Source: CAD feature listing. Evaluate the final solid. Frame: model axes, mm. Face numbers are marked on the shaded views. A direction names the side the tool comes from. Coordinates: 2 decimals unless noted, no trailing zeros. Write each loop counter-clockwise with the first axis right and the second up, starting at its lowest first coordinate (ties: lowest second). Pieces come first, ordered by that corner, then holes. Notation, with made-up numbers: (-20.75, -15) - (31.25, -15) arc R7 ccw to (31.25, -11) - close; hole circle Ø3 at (4, 31.5). An arc over 180 degrees is marked (long way). One line per item, written item: value.
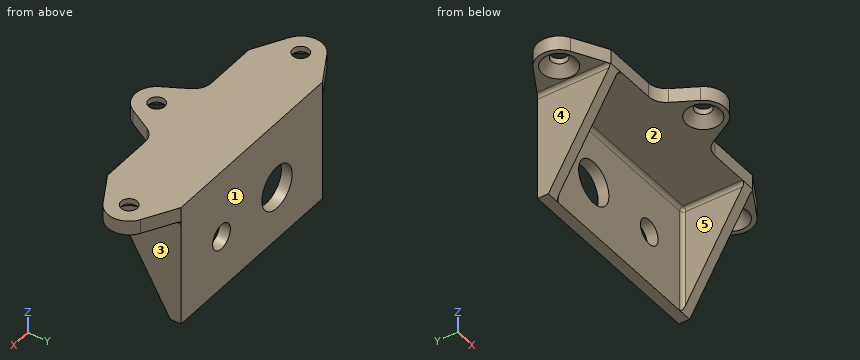
from build123d import *

# Parameters (mm, degrees)
SKETCH1_W                                       = 50
SKETCH1_H                                       = 30
SKETCH1_R                                       = 6
SKETCH1_R_2                                     = 3.5
BOSS_EXTRUDE1_DEPTH                             = 3
SKETCH2_W                                       = 50
SKETCH2_H                                       = 20.5
BOSS_EXTRUDE2_DEPTH                             = 4
BOSS_EXTRUDE3_DEPTH                             = 3
BOSS_EXTRUDE4_START                             = -50
BOSS_EXTRUDE4_DEPTH                             = 3
BOSS_EXTRUDE5_DEPTH                             = 4
CSK_FOR_M4_FLAT_HEAD_MACHINE_SCREW1_D           = 4.5
CSK_FOR_M4_FLAT_HEAD_MACHINE_SCREW1_DEPTH       = 10
CSK_FOR_M4_FLAT_HEAD_MACHINE_SCREW1_CSINK_D     = 9.4
CSK_FOR_M4_FLAT_HEAD_MACHINE_SCREW1_CSINK_ANGLE = 90
CSK_FOR_M4_FLAT_HEAD_MACHINE_SCREW1_TIP         = 1.351936393
FILLET1_R                                       = 5
FILLET2_R                                       = 1


with BuildPart() as part:
    # Sketch1 → Boss-Extrude1 (new body)
    with BuildSketch(Plane(origin=(0, 0, 0), x_dir=(1, 0, 0), z_dir=(0, 1, 0))):
        Rectangle(SKETCH1_W, SKETCH1_H)
        with Locations(Location((-10, 0, 0), (0, 0, 270))):
            Circle(SKETCH1_R, mode=Mode.SUBTRACT)
        with Locations(Location((12, 0, 0), (0, 0, 270))):
            Circle(SKETCH1_R_2, mode=Mode.SUBTRACT)
    extrude(amount=BOSS_EXTRUDE1_DEPTH)

    # Sketch2 → Boss-Extrude2 (add)
    with BuildSketch(Plane.XY.offset(15)):
        with Locations((0, -7.25)):
            Rectangle(SKETCH2_W, SKETCH2_H)
    extrude(amount=BOSS_EXTRUDE2_DEPTH)

    # Sketch3 → Boss-Extrude3 (add)
    with BuildSketch(Plane.ZY.offset(25)):
        Polygon((-15, 3), (-15, 0), (15, -17.5), (19, -17.5), (19, 3), align=None)
    extrude(amount=BOSS_EXTRUDE3_DEPTH)

    # Sketch3<2> → Boss-Extrude4 (add)
    with BuildSketch(Plane.ZY.offset(25).offset(BOSS_EXTRUDE4_START)):
        Polygon((-15, 3), (-15, 0), (15, -17.5), (19, -17.5), (19, 3), align=None)
    extrude(amount=-BOSS_EXTRUDE4_DEPTH)

    # Sketch5 → Boss-Extrude5 (add)
    with BuildSketch(Plane.XY.offset(19)):
        with BuildLine():
            Line((-28, 3), (-36.937527692, -2.018276473))
            ThreePointArc((-36.937527692, -2.018276473), (-40, -7.25), (-36.937527692, -12.481723527))
            Line((-36.937527692, -12.481723527), (-28, -17.5))
            Line((-28, -17.5), (-28, 3))
        make_face()
        with BuildLine():
            Line((28, 3), (36.937527692, -2.018276473))
            ThreePointArc((36.937527692, -2.018276473), (40, -7.25), (36.937527692, -12.481723527))
            Line((36.937527692, -12.481723527), (28, -17.5))
            Line((28, -17.5), (28, 3))
        make_face()
        with BuildLine():
            Line((10.25, -17.5), (-10.25, -17.5))
            Line((-10.25, -17.5), (-5.231723527, -26.437527692))
            ThreePointArc((-5.231723527, -26.437527692), (0, -29.5), (5.231723527, -26.437527692))
            Line((5.231723527, -26.437527692), (10.25, -17.5))
        make_face()
    extrude(amount=-BOSS_EXTRUDE5_DEPTH)

    # CSK for M4 Flat Head Machine Screw1
    with Locations(Plane(origin=(0, 0, 15), x_dir=(-1, 0, 0), z_dir=(0, 0, -1))):
        with Locations((-34, -7.25), (34, -7.25), (0, -23.5)):
            CounterSinkHole(CSK_FOR_M4_FLAT_HEAD_MACHINE_SCREW1_D / 2, CSK_FOR_M4_FLAT_HEAD_MACHINE_SCREW1_CSINK_D / 2, depth=CSK_FOR_M4_FLAT_HEAD_MACHINE_SCREW1_DEPTH, counter_sink_angle=CSK_FOR_M4_FLAT_HEAD_MACHINE_SCREW1_CSINK_ANGLE)
            with Locations((0, 0, -(CSK_FOR_M4_FLAT_HEAD_MACHINE_SCREW1_DEPTH + CSK_FOR_M4_FLAT_HEAD_MACHINE_SCREW1_TIP / 2))):  # 118° drill point
                Cone(0, CSK_FOR_M4_FLAT_HEAD_MACHINE_SCREW1_D / 2, CSK_FOR_M4_FLAT_HEAD_MACHINE_SCREW1_TIP, mode=Mode.SUBTRACT)

    # Fillet1
    fillet1_edges = [part.edges().sort_by_distance(p)[0] for p in [
        (-10.25, -17.5, 17),
        (10.25, -17.5, 17),
    ]]
    fillet(fillet1_edges, radius=FILLET1_R)

    # Fillet2
    # the kernel refuses this fillet: 1 mm, written as the material it adds along each edge
    with BuildSketch(Plane(origin=(-24, -1, 14), x_dir=(0, 1, 0), z_dir=(0, 0, 1))) as fillet2_piece_1_section:
        Polygon((0, 0), (FILLET2_R, 0), (FILLET2_R, FILLET2_R), (0, FILLET2_R), align=None)
    fillet2_piece_1 = extrude(amount=FILLET2_R, mode=Mode.PRIVATE)
    fillet2_piece_1 = fillet2_piece_1 - Plane(origin=(-24, -1, 14), x_dir=(0.7071067811865475, -0.7071067811865475, 0), z_dir=(0, 0, 1)) * Sphere(FILLET2_R, mode=Mode.PRIVATE)
    add(fillet2_piece_1)
    with BuildSketch(Plane(origin=(24, -1, 14), x_dir=(1, 0, 0), z_dir=(0, 0, 1))) as fillet2_piece_2_section:
        Polygon((0, 0), (FILLET2_R, 0), (FILLET2_R, FILLET2_R), (0, FILLET2_R), align=None)
    fillet2_piece_2 = extrude(amount=FILLET2_R, mode=Mode.PRIVATE)
    fillet2_piece_2 = fillet2_piece_2 - Plane(origin=(24, -1, 14), x_dir=(-0.7071067811865475, -0.7071067811865475, 0), z_dir=(0, 0, 1)) * Sphere(FILLET2_R, mode=Mode.PRIVATE)
    add(fillet2_piece_2)
    with BuildSketch(Plane(origin=(-25, -17.5, 15), x_dir=(1, 0, 0), z_dir=(0, 1, 0))) as fillet2_piece_3_section:
        with BuildLine():
            CenterArc((FILLET2_R, FILLET2_R), FILLET2_R, 180, 90)
            Line((0, FILLET2_R), (0, 0))
            Line((0, 0), (FILLET2_R, 0))
        make_face()
    fillet2_piece_3 = extrude(amount=16.5, mode=Mode.PRIVATE)
    fillet2_piece_3 = split(fillet2_piece_3, bisect_by=Plane(origin=(-24.77263385, -15.290921561, 11.213008391), z_dir=(0, 0.8637789008984336, 0.5038710255240861)), keep=Keep.TOP, mode=Mode.PRIVATE)
    add(fillet2_piece_3)
    with BuildSketch(Plane(origin=(25, -1, 15), x_dir=(-1, 0, 0), z_dir=(0, -1, 0))) as fillet2_piece_4_section:
        with BuildLine():
            CenterArc((FILLET2_R, FILLET2_R), FILLET2_R, 180, 90)
            Line((0, FILLET2_R), (0, 0))
            Line((0, 0), (FILLET2_R, 0))
        make_face()
    fillet2_piece_4 = extrude(amount=16.5, mode=Mode.PRIVATE)
    fillet2_piece_4 = split(fillet2_piece_4, bisect_by=Plane(origin=(24.77263385, -15.290921561, 11.213008391), z_dir=(0, 0.8637789008984336, 0.5038710255240861)), keep=Keep.TOP, mode=Mode.PRIVATE)
    add(fillet2_piece_4)
    with BuildSketch(Plane(origin=(24, 0, 15), x_dir=(0, -1, 0), z_dir=(-1, 0, 0))) as fillet2_piece_5:
        with BuildLine():
            CenterArc((FILLET2_R, -FILLET2_R), FILLET2_R, 90, 90)
            Line((0, -FILLET2_R), (0, 0))
            Line((0, 0), (FILLET2_R, 0))
        make_face()
    extrude(amount=48)
    with BuildSketch(Plane(origin=(-25, 0, 14), x_dir=(1, 0, 0), z_dir=(0, 0, -1))) as fillet2_piece_6_section:
        with BuildLine():
            CenterArc((FILLET2_R, FILLET2_R), FILLET2_R, 180, 90)
            Line((0, FILLET2_R), (0, 0))
            Line((0, 0), (FILLET2_R, 0))
        make_face()
    fillet2_piece_6 = extrude(amount=29, mode=Mode.PRIVATE)
    fillet2_piece_6 = split(fillet2_piece_6, bisect_by=Plane(origin=(-24.77197237, -6.451381469, -3.94048891), z_dir=(0, 0.8637789008984336, 0.5038710255240861)), keep=Keep.TOP, mode=Mode.PRIVATE)
    add(fillet2_piece_6)
    with BuildSketch(Plane(origin=(25, 0, -15), x_dir=(0, -1, 0), z_dir=(0, 0, 1))) as fillet2_piece_7_section:
        with BuildLine():
            CenterArc((FILLET2_R, -FILLET2_R), FILLET2_R, 90, 90)
            Line((0, -FILLET2_R), (0, 0))
            Line((0, 0), (FILLET2_R, 0))
        make_face()
    fillet2_piece_7 = extrude(amount=29, mode=Mode.PRIVATE)
    fillet2_piece_7 = split(fillet2_piece_7, bisect_by=Plane(origin=(24.77197237, -6.451381469, -3.94048891), z_dir=(0, 0.8637789008984336, 0.5038710255240861)), keep=Keep.TOP, mode=Mode.PRIVATE)
    add(fillet2_piece_7)
    with BuildSketch(Plane(origin=(-28, -20, 15), x_dir=(0, 0, -1), z_dir=(0, 1, 0))) as fillet2_piece_8_section:
        with BuildLine():
            CenterArc((FILLET2_R, FILLET2_R), FILLET2_R, 180, 90)
            Line((0, FILLET2_R), (0, 0))
            Line((0, 0), (FILLET2_R, 0))
        make_face()
    fillet2_piece_8 = extrude(amount=23, mode=Mode.PRIVATE)
    fillet2_piece_8 = split(fillet2_piece_8, bisect_by=Plane(origin=(-28.224621948, -14.787732132, 10.350397941), z_dir=(0, 0.8637789008984336, 0.5038710255240861)), keep=Keep.TOP, mode=Mode.PRIVATE)
    fillet2_piece_8 = split(fillet2_piece_8, bisect_by=Plane(origin=(-32.565520465, -14.936534495, 14.773416923), z_dir=(0.48958794860434196, 0.8719539211342491, 0)), keep=Keep.TOP, mode=Mode.PRIVATE)
    fillet2_piece_8 = split(fillet2_piece_8, bisect_by=Plane(origin=(-32.527453001, 0.457908757, 14.773416923), z_dir=(0.48958794860434235, -0.8719539211342491, 0)), keep=Keep.TOP, mode=Mode.PRIVATE)
    add(fillet2_piece_8)
    with BuildSketch(Plane(origin=(28, -20, 15), x_dir=(1, 0, 0), z_dir=(0, 1, 0))) as fillet2_piece_9_section:
        with BuildLine():
            CenterArc((FILLET2_R, FILLET2_R), FILLET2_R, 180, 90)
            Line((0, FILLET2_R), (0, 0))
            Line((0, 0), (FILLET2_R, 0))
        make_face()
    fillet2_piece_9 = extrude(amount=23, mode=Mode.PRIVATE)
    fillet2_piece_9 = split(fillet2_piece_9, bisect_by=Plane(origin=(32.565520464, -14.936534495, 14.773416923), z_dir=(-0.48958794860434196, 0.8719539211342491, 0)), keep=Keep.TOP, mode=Mode.PRIVATE)
    fillet2_piece_9 = split(fillet2_piece_9, bisect_by=Plane(origin=(28.224621948, -14.787732132, 10.350397941), z_dir=(0, 0.8637789008984336, 0.5038710255240861)), keep=Keep.TOP, mode=Mode.PRIVATE)
    fillet2_piece_9 = split(fillet2_piece_9, bisect_by=Plane(origin=(32.527453001, 0.457908757, 14.773416923), z_dir=(-0.48958794860434235, -0.8719539211342491, 0)), keep=Keep.TOP, mode=Mode.PRIVATE)
    add(fillet2_piece_9)


solid = part.part
1) Section query B-B on x = 12. Output: boundary loops of the cut face in (y, z).
Values found:
outline: (-17.64, 15) - (-1, 15) arc R1 cw to (0, 14) - (0, 3.5) - (3, 3.5) - (3, 19) - (-17.64, 19) - close; (0, -15) - (3, -15) - (3, -3.5) - (0, -3.5) - close
2) Section query C-C on y = -23.5. Output: boundary loops of the cut face in (x, z).
Values found:
outline: (-6.88, 15) - (-4.7, 15) - (-2.25, 17.45) - (-2.25, 19) - (-6.88, 19) - close; (2.25, 17.45) - (4.7, 15) - (6.88, 15) - (6.88, 19) - (2.25, 19) - close
3) Section query A-A on z = 0. Output: boundary loops of the cut face in (x, y).
Values found:
outline: (-28, -8.75) - (-25, -8.75) - (-25, -1) arc R1 cw to (-24, 0) - (-16, 0) - (-16, 3) - (-28, 3) - close; (-4, 0) - (8.5, 0) - (8.5, 3) - (-4, 3) - close; (15.5, 0) - (24, 0) arc R1 cw to (25, -1) - (25, -8.75) - (28, -8.75) - (28, 3) - (15.5, 3) - close
4) Material intervals for line 1 (X direction, y = -7.25, z = 18.2); line 2 (X direction, y = -1.5, z = -4.5); line 3 (Y direction, x = 0, z = 18.2), sorted ascending.
Values found:
line 1: -40 to -36.25, -31.75 to 31.75, 36.25 to 40
line 2: -28 to -25, 25 to 28
line 3: -29.5 to -25.75, -21.25 to 3
5) Contact query for flat-ended pins moving along their axis: P1, Ø4, axis at x = 23.5, z = -5, coming from the -Y side (3 decimals); P2, Ø10, axis at x = 7, y = -8, coming from the -Z side; P3, Ø3, axis at x = 22.5, z = 16.5, coming from the -Y side. Output: stop coordinate, or through.
Values found:
P1: y = -6.605
P2: z = 15
P3: y = -17.5
6) Draft query along X for the marked faces 3, 4 and 5. Return one class per face: released by +X, released by -X, zero draft, split by the parting line, or undercut.
Values found:
face 3: released by +X
face 4: released by -X
face 5: undercut
7) Reachability of the marked faces 1 and 2 from +Z, -Z, +X, -X, +Y, -Y: full face, straight path, thin tool, end or side. Return the list, or none.
Values found:
face 1: +Z, -Z, +X, -X, +Y
face 2: -Z, -Y
8) Section query D-D on y = -7.25. Output: boundary loops of the cut face in (x, z), then the cut area to 3 significant figures.
Values found:
outline: (-40, 15) - (-38.7, 15) - (-36.25, 17.45) - (-36.25, 19) - (-40, 19) - close; (-31.75, 17.45) - (-29.3, 15) - (-29, 15) arc R1 cw to (-28, 14) - (-28, -2.57) - (-25, -2.57) - (-25, 14) arc R1 cw to (-24, 15) - (24, 15) arc R1 cw to (25, 14) - (25, -2.57) - (28, -2.57) - (28, 14) arc R1 cw to (29, 15) - (29.3, 15) - (31.75, 17.45) - (31.75, 19) - (-31.75, 19) - close; (36.25, 17.45) - (38.7, 15) - (40, 15) - (40, 19) - (36.25, 19) - close
area: 378 mm2
